Could you check a few things on this model? Use its own coordinates, in mm. Round coordinates to 2 decimals unless told otherwise and drop trailing zeros. Write each loop counter-clockwise with the first axis right and the second up, starting at its lowest first coordinate (ties: lowest second). Pieces come first, ordered by that corner, then holes. Notation, with made-up numbers: (-3, -9.75) -> (22, -9.75) arc R27 ccw to (22, 22.25) -> close; hole circle Ø8 at (32.5, -29). An arc over 180 degrees is marked (long way). Return JSON: item names as keys, results as strings.
from build123d import *

# Parameters (mm, degrees)
SALIENTE_EXTRUIR1_DEPTH = 5


with BuildPart() as part:
    # Croquis1 → Saliente-Extruir1 (new body)
    with BuildSketch(Plane.XY):
        with BuildLine():
            Line((87.636038969, 36.121320344), (116.796683693, 6.96067562))
            Line((116.796683693, 6.96067562), (116.796683693, 0))
            Line((116.796683693, 0), (0, 0))
            Line((0, 0), (0, 34))
            ThreePointArc((0, 34), (0.878679656, 36.121320344), (3, 37))
            Line((3, 37), (85.514718626, 37))
            ThreePointArc((85.514718626, 37), (86.662768923, 36.771638598), (87.636038969, 36.121320344))
        make_face()
    extrude(amount=SALIENTE_EXTRUIR1_DEPTH)


solid = part.part
1) I want a section at A-A, the plane z = 2.75. Please give me the cut outline in (x, y), and give its area (3 significant figures).
Return value:
{"outline": "(0, 0) -> (116.8, 0) -> (116.8, 6.96) -> (87.64, 36.12) arc R3 ccw to (85.51, 37) -> (3, 37) arc R3 ccw to (0, 34) -> close", "area": "3,870 mm²"}
2) Thinking about a two-plate mould opening in Z: for faces 1 (the face through (86.648, 36.778, 2.465)), 2 (the face through (59, 19, 0)), 3 (the face through (59, 19, 5)), which applies, pulls with the +Z half, pulls with the -Z half, needs draft (parallel to the pull), parting line crosses it, or undercut?
Return value:
{"face 1": "needs draft", "face 2": "pulls with the -Z half", "face 3": "pulls with the +Z half"}
3) I want a section at C-C, the plane x = 104.5. Please give me the cut outline in (y, z), and give its area (3 significant figures).
Return value:
{"outline": "(0, 0) -> (19.26, 0) -> (19.26, 5) -> (0, 5) -> close", "area": "96.3 mm²"}
4) I want a section at B-B, the plane y = 17.5. Please give me the cut outline in (x, z), and give its area (3 significant figures).
Return value:
{"outline": "(0, 0) -> (106.26, 0) -> (106.26, 5) -> (0, 5) -> close", "area": "531 mm²"}
5) If I drill on probe 1 along X at (y, z) = (25.5, 4.5); probe 2 along X at (y, z) = (19.5, 2.3); probe 3 along Y at (x, z) = (90.5, 3.05), over which ranges is the centre line in solid material (lowest first)? Write a range as [from, to].
Return value:
{"probe 1": "[0, 98.26]", "probe 2": "[0, 104.26]", "probe 3": "[0, 33.26]"}
